Here's how the part is built. I have some questions about the finished solid (model axes, mm). A direction names the side the tool comes from. Give positions to 0.01 mm unless a question says otherwise; leave off trailing zeros. Write each loop counter-clockwise with the first axis right and the second up, starting at its lowest first coordinate (ties: lowest second). Pieces come first, ordered by that corner, then holes. Notation, with made-up numbers: (-16, 4.25) -> (30, 4.25) arc R22 cw to (30, 21.25) -> close; hole circle Ø5 at (-12.5, 19). An arc over 180 degrees is marked (long way). Use CSV: the item, a comma, the result in double quotes. Start each with the question number.
(1) Suppose I cut it at A-A on z = 11.25. List the corners of the cut face in (x, y) for me.
(2) If we mould it in two halves opening along Y, with no side actions, what happens to faces 4 (the flat face through (5.7, 50, -0.3)), 5 (the flat face through (19.59, 24.65, 0.35)), 6 (the cylindrical face through (27.031, 38.137, 16.479))? For each: pulls with the +Y half, pulls with the -Y half, needs draft (parallel to the pull), parting line crosses it, or undercut.
(3) I need wall thicknesses on L1, parallel to X at y = 34, z = 7.5; L2, parallel to Z at x = 14, y = 6; L3, parallel to Z at x = 29.5, y = 32. Which ranges of each line are inside material? Lowest first, please. Write a range as [from, to].
(4) Suppose I cut it at C-C on y = 26. List the corners of the cut face in (x, z) for me.
(5) Suppose I cut it at B-B on x = 27. List the corners of the cut face in (y, z) for me, plus the area to 3 significant figures.
(6) Suppose I cut it at D-D on y = 11. Give the number of separate pieces and of enclosed holes in the cut face, plus the area to 3 significant figures.
(7) Which directions (+Z, -Z, +X, -X, +Y, -Y) give clear straight access to the entire face, cutting with the end or side of a thin tool? Please do faces 1 (the cylindrical face through (-6.07, 24.65, 16.88)), 2 (the flat face through (-8, 25, 10)), 3 (the flat face through (-13, 25, 18)).
(8) For pin 1 Ø10 at (y, z) = (27, 8) entering from +X; pin 2 Ø10 at (x, y) = (29.5, 18.5) entering from -Z; pin 3 Ø7 at (y, z) = (35.5, 9.5) entering from -X, each with a flat end and sliding along its axis, tell me the tip position at first contact or that it passes through.
from build123d import *

# Parameters (mm, degrees)
SKETCH1_W                      = 15
SKETCH1_H                      = 50
BASE_FLANGE1_DEPTH             = 3
EDGE_FLANGE5_STRIP_CUT_DEPTH   = 50
EDGE_FLANGE5_STRIP_CUT_2_DEPTH = 50
EDGE_FLANGE5_DEPTH             = 50
EDGE_FLANGE5_BEND_DEPTH        = 50
EDGE_FLANGE6_STRIP_CUT_DEPTH   = 50
EDGE_FLANGE6_STRIP_CUT_2_DEPTH = 50
EDGE_FLANGE6_DEPTH             = 50
EDGE_FLANGE6_BEND_DEPTH        = 50
EDGE_FLANGE7_STRIP_W           = 13.4732
EDGE_FLANGE7_STRIP_H           = 3
EDGE_FLANGE7_STRIP_CUT_DEPTH   = 50
EDGE_FLANGE7_STRIP_2_W         = 13.4732
EDGE_FLANGE7_STRIP_2_H         = 3
EDGE_FLANGE7_STRIP_CUT_2_DEPTH = 50
EDGE_FLANGE7_DEPTH             = 50
EDGE_FLANGE7_BEND_DEPTH        = 50
TAP_DRILL_FOR_M5X0_8_TAP1_D    = 4.2


# Sheet-metal steps are written as plain solids
with BuildPart() as part:
    # Sketch1 → Base-Flange1 (new body)
    with BuildSketch(Plane.XY):
        with Locations((7.5, 25)):
            Rectangle(SKETCH1_W, SKETCH1_H)
    extrude(amount=-BASE_FLANGE1_DEPTH)

    # Edge-Flange5 strip (across the edge) → Edge-Flange5 strip cut (cut)
    with BuildSketch(Plane(origin=(15, 0, 0), x_dir=(-0.7071067811865438, 0, 0.7071067811865512), z_dir=(0, 1, 0))):
        Polygon((-11.432566283, 7.189925596), (-1.905575199, -2.337065489), (0.215745145, -0.215745145), (-9.311245939, 9.311245939), align=None)
    extrude(amount=EDGE_FLANGE5_STRIP_CUT_DEPTH, mode=Mode.SUBTRACT)

    # Edge-Flange5 strip 2 (across the edge) → Edge-Flange5 strip cut 2 (cut)
    with BuildSketch(Plane(origin=(0, 50, 0), x_dir=(0.7071067811865438, 0, 0.7071067811865512), z_dir=(0, -1, 0))):
        Polygon((-11.432566283, 7.189925596), (-1.905575199, -2.337065489), (0.215745145, -0.215745145), (-9.311245939, 9.311245939), align=None)
    extrude(amount=EDGE_FLANGE5_STRIP_CUT_2_DEPTH, mode=Mode.SUBTRACT)

    # Edge-Flange5 section (across the edge) → Edge-Flange5 (add)
    with BuildSketch(Plane(origin=(15, 0, 0), x_dir=(-0.7071067811865438, 0, 0.7071067811865512), z_dir=(0, 1, 0))):
        with BuildLine():
            Line((-3, 0.30510971), (-3, 7.071))
            Line((-3, 7.071), (0, 7.071))
            Line((0, 7.071), (0, 0.30510971))
            ThreePointArc((0, 0.30510971), (0.056070336, 0.023225094), (0.215745145, -0.215745145))
            Line((0.215745145, -0.215745145), (-1.905575199, -2.337065489))
            ThreePointArc((-1.905575199, -2.337065489), (-2.715568261, -1.124825203), (-3, 0.30510971))
        make_face()
    extrude(amount=EDGE_FLANGE5_DEPTH)

    # Edge-Flange5 section 2 (across the edge) → Edge-Flange5 bend (add)
    with BuildSketch(Plane(origin=(0, 50, 0), x_dir=(0.7071067811865438, 0, 0.7071067811865512), z_dir=(0, -1, 0))):
        with BuildLine():
            Line((-3, 0.30510971), (-3, 7.071))
            Line((-3, 7.071), (0, 7.071))
            Line((0, 7.071), (0, 0.30510971))
            ThreePointArc((0, 0.30510971), (0.056070336, 0.023225094), (0.215745145, -0.215745145))
            Line((0.215745145, -0.215745145), (-1.905575199, -2.337065489))
            ThreePointArc((-1.905575199, -2.337065489), (-2.715568261, -1.124825203), (-3, 0.30510971))
        make_face()
    extrude(amount=EDGE_FLANGE5_BEND_DEPTH)

    # Edge-Flange6 strip (across the edge) → Edge-Flange6 strip cut (cut)
    with BuildSketch(Plane(origin=(-4.99995205, 50, 4.99995205), x_dir=(1, 0, 0), z_dir=(0, -1, 0))):
        Polygon((-11.432566283, 7.189925596), (-1.905575199, -2.337065489), (0.215745145, -0.215745145), (-9.311245939, 9.311245939), align=None)
    extrude(amount=EDGE_FLANGE6_STRIP_CUT_DEPTH, mode=Mode.SUBTRACT)

    # Edge-Flange6 strip 2 (across the edge) → Edge-Flange6 strip cut 2 (cut)
    with BuildSketch(Plane(origin=(19.99995205, 0, 4.99995205), x_dir=(-1, 0, 0), z_dir=(0, 1, 0))):
        Polygon((-11.432566283, 7.189925596), (-1.905575199, -2.337065489), (0.215745145, -0.215745145), (-9.311245939, 9.311245939), align=None)
    extrude(amount=EDGE_FLANGE6_STRIP_CUT_2_DEPTH, mode=Mode.SUBTRACT)

    # Edge-Flange6 section (across the edge) → Edge-Flange6 (add)
    with BuildSketch(Plane(origin=(-4.99995205, 50, 4.99995205), x_dir=(1, 0, 0), z_dir=(0, -1, 0))):
        with BuildLine():
            Line((-3, 0.30510971), (-3, 10))
            Line((-3, 10), (0, 10))
            Line((0, 10), (0, 0.30510971))
            ThreePointArc((0, 0.30510971), (0.056070336, 0.023225094), (0.215745145, -0.215745145))
            Line((0.215745145, -0.215745145), (-1.905575199, -2.337065489))
            ThreePointArc((-1.905575199, -2.337065489), (-2.715568261, -1.124825203), (-3, 0.30510971))
        make_face()
    extrude(amount=EDGE_FLANGE6_DEPTH)

    # Edge-Flange6 section 2 (across the edge) → Edge-Flange6 bend (add)
    with BuildSketch(Plane(origin=(19.99995205, 0, 4.99995205), x_dir=(-1, 0, 0), z_dir=(0, 1, 0))):
        with BuildLine():
            Line((-3, 0.30510971), (-3, 10))
            Line((-3, 10), (0, 10))
            Line((0, 10), (0, 0.30510971))
            ThreePointArc((0, 0.30510971), (0.056070336, 0.023225094), (0.215745145, -0.215745145))
            Line((0.215745145, -0.215745145), (-1.905575199, -2.337065489))
            ThreePointArc((-1.905575199, -2.337065489), (-2.715568261, -1.124825203), (-3, 0.30510971))
        make_face()
    extrude(amount=EDGE_FLANGE6_BEND_DEPTH)

    # Edge-Flange7 strip (across the edge) → Edge-Flange7 strip cut (cut)
    with BuildSketch(Plane(origin=(-7.99995205, 0, 14.99995205), x_dir=(0, 0, -1), z_dir=(0, 1, 0))):
        with Locations((-6, -1.5)):
            Rectangle(EDGE_FLANGE7_STRIP_W, EDGE_FLANGE7_STRIP_H)
    extrude(amount=EDGE_FLANGE7_STRIP_CUT_DEPTH, mode=Mode.SUBTRACT)

    # Edge-Flange7 strip 2 (across the edge) → Edge-Flange7 strip cut 2 (cut)
    with BuildSketch(Plane(origin=(22.99995205, 50, 14.99995205), x_dir=(0, 0, -1), z_dir=(0, -1, 0))):
        with Locations((-6, -1.5)):
            Rectangle(EDGE_FLANGE7_STRIP_2_W, EDGE_FLANGE7_STRIP_2_H)
    extrude(amount=EDGE_FLANGE7_STRIP_CUT_2_DEPTH, mode=Mode.SUBTRACT)

    # Edge-Flange7 section (across the edge) → Edge-Flange7 (add)
    with BuildSketch(Plane(origin=(-7.99995205, 0, 14.99995205), x_dir=(0, 0, -1), z_dir=(0, 1, 0))):
        with BuildLine():
            Line((-3, 0.7366), (-3, 10))
            Line((-3, 10), (0, 10))
            Line((0, 10), (0, 0.7366))
            ThreePointArc((0, 0.7366), (0.215745145, 0.215745145), (0.7366, 0))
            Line((0.7366, 0), (0.7366, -3))
            ThreePointArc((0.7366, -3), (-1.905575199, -1.905575199), (-3, 0.7366))
        make_face()
    extrude(amount=EDGE_FLANGE7_DEPTH)

    # Edge-Flange7 section 2 (across the edge) → Edge-Flange7 bend (add)
    with BuildSketch(Plane(origin=(22.99995205, 50, 14.99995205), x_dir=(0, 0, -1), z_dir=(0, -1, 0))):
        with BuildLine():
            Line((-3, 0.7366), (-3, 10))
            Line((-3, 10), (0, 10))
            Line((0, 10), (0, 0.7366))
            ThreePointArc((0, 0.7366), (0.215745145, 0.215745145), (0.7366, 0))
            Line((0.7366, 0), (0.7366, -3))
            ThreePointArc((0.7366, -3), (-1.905575199, -1.905575199), (-3, 0.7366))
        make_face()
    extrude(amount=EDGE_FLANGE7_BEND_DEPTH)

    # Tap Drill for M5x0.8 Tap1 (through all)
    with Locations(Plane.XY.offset(17.99995205)):
        with Locations((-12.99995205, 10), (-12.99995205, 40), (27.99995205, 10), (27.99995205, 40)):
            Hole(TAP_DRILL_FOR_M5X0_8_TAP1_D / 2)


solid = part.part
Geometry says:
1,outline,"(-8, 0) -> (-5, 0) -> (-5, 50) -> (-8, 50) -> close; (20, 0) -> (23, 0) -> (23, 50) -> (20, 50) -> close"
2,face 4,"pulls with the +Y half"
2,face 5,"needs draft"
2,face 6,"undercut"
3,L1,"[-8, -5], [20, 23]"
3,L2,"[-3, 0]"
3,L3,"[15, 18]"
4,outline,"(-18, 15) -> (-8.74, 15) arc R0.74 cw to (-8, 14.26) -> (-8, 5.31) arc R3.74 ccw to (-6.91, 2.66) -> (-2.34, -1.91) arc R3.74 ccw to (0.31, -3) -> (14.69, -3) arc R3.74 ccw to (17.34, -1.91) -> (21.91, 2.66) arc R3.74 ccw to (23, 5.31) -> (23, 14.26) arc R0.74 cw to (23.74, 15) -> (33, 15) -> (33, 18) -> (23.74, 18) arc R3.74 ccw to (20, 14.26) -> (20, 5.31) arc R0.74 cw to (19.78, 4.78) -> (15.22, 0.22) arc R0.74 cw to (14.69, 0) -> (0.31, 0) arc R0.74 cw to (-0.22, 0.22) -> (-4.78, 4.78) arc R0.74 cw to (-5, 5.31) -> (-5, 14.26) arc R3.74 ccw to (-8.74, 18) -> (-18, 18) -> close"
5,outline,"(0, 15) -> (8.15, 15) -> (8.15, 18) -> (0, 18) -> close; (11.85, 15) -> (38.15, 15) -> (38.15, 18) -> (11.85, 18) -> close; (41.85, 15) -> (50, 15) -> (50, 18) -> (41.85, 18) -> close"
5,area,"128 mm²"
6,separate pieces,"3"
6,enclosed holes,"0"
6,area,"211 mm²"
7,face 1,"+Z, +Y, -Y"
7,face 2,"-Z, -X, +Y, -Y"
7,face 3,"+Z, +X, -X, +Y, -Y"
8,pin 1,"x = 23"
8,pin 2,"z = 15"
8,pin 3,"x = -8"
